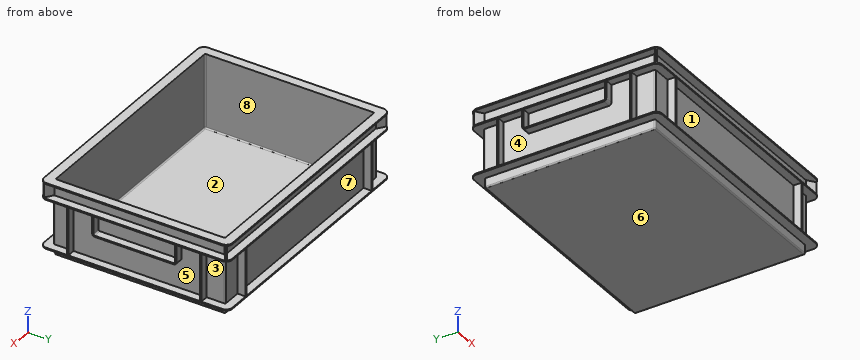
from build123d import *

# Parameters (mm, degrees)
F0_W      = 372
F0_H      = 272
F1_DEPTH  = 15
F2_W      = 372
F2_H      = 272
F3_DEPTH  = 2
F5_DEPTH  = 76
F7_DEPTH  = 2
F9_DEPTH  = 23
F11_DEPTH = 2
F12_W     = 370
F12_H     = 270
F13_DEPTH = 118
F15_DEPTH = 13
F17_DEPTH = 13
F18_R     = 2


with BuildPart() as f1:
    # F0 (on Top) → F1 (new body)
    with BuildSketch(Plane.XY):
        Rectangle(F0_W, F0_H)
    extrude(amount=F1_DEPTH)

    # F2 (on face) → F3 (join)
    with BuildSketch(Plane.XY.offset(15)):
        with BuildLine():
            Line((-190, -150), (190, -150))
            ThreePointArc((190, -150), (197.0710678119, -147.0710678119), (200, -140))
            Line((200, -140), (200, 140))
            ThreePointArc((200, 140), (197.0710678119, 147.0710678119), (190, 150))
            Line((190, 150), (-190, 150))
            ThreePointArc((-190, 150), (-197.0710678119, 147.0710678119), (-200, 140))
            Line((-200, 140), (-200, -140))
            ThreePointArc((-200, -140), (-197.0710678119, -147.0710678119), (-190, -150))
        make_face()
        Rectangle(F2_W, F2_H, mode=Mode.SUBTRACT)
        Rectangle(F2_W, F2_H)
    extrude(amount=F3_DEPTH)

    # F4 (on face) → F5 (join)
    with BuildSketch(Plane.XY.offset(17)):
        Polygon((157, -137), (187, -137), (187, -107), (200, -107), (200, -105), (187, -105), (187, 105), (200, 105), (200, 107), (187, 107), (187, 137), (157, 137), (157, 150), (155, 150), (155, 137), (-155, 137), (-155, 150), (-157, 150), (-157, 137), (-187, 137), (-187, 107), (-200, 107), (-200, 105), (-187, 105), (-187, -105), (-200, -105), (-200, -107), (-187, -107), (-187, -137), (-157, -137), (-157, -150), (-155, -150), (-155, -137), (155, -137), (155, -150), (157, -150), align=None)
    extrude(amount=F5_DEPTH)

    # F6 (on face) → F7 (join)
    with BuildSketch(Plane.XY.offset(93)):
        with BuildLine():
            Line((190, 150), (-190, 150))
            ThreePointArc((-190, 150), (-197.0710678119, 147.0710678119), (-200, 140))
            Line((-200, 140), (-200, -140))
            ThreePointArc((-200, -140), (-197.0710678119, -147.0710678119), (-190, -150))
            Line((-190, -150), (190, -150))
            ThreePointArc((190, -150), (197.0710678119, -147.0710678119), (200, -140))
            Line((200, -140), (200, 140))
            ThreePointArc((200, 140), (197.0710678119, 147.0710678119), (190, 150))
        make_face()
    extrude(amount=F7_DEPTH)

    # F8 (on face) → F9 (join)
    with BuildSketch(Plane.XY.offset(95)):
        with BuildLine():
            Line((-185.3079227659, -137), (185.3079227659, -137))
            Line((185.3079227659, -137), (197.8531877713, -146.1909160735))
            ThreePointArc((197.8531877713, -146.1909160735), (198.4340605379, -145.3727667773), (198.9300207482, -144.5005254622))
            Line((198.9300207482, -144.5005254622), (187, -135.7603498338))
            Line((187, -135.7603498338), (187, 135.7603498338))
            Line((187, 135.7603498338), (198.9300207482, 144.5005254622))
            ThreePointArc((198.9300207482, 144.5005254622), (198.4340605379, 145.3727667773), (197.8531877713, 146.1909160735))
            Line((197.8531877713, 146.1909160735), (185.3079227659, 137))
            Line((185.3079227659, 137), (-185.3079227659, 137))
            Line((-185.3079227659, 137), (-197.8531877713, 146.1909160735))
            ThreePointArc((-197.8531877713, 146.1909160735), (-198.4340605379, 145.3727667773), (-198.9300207482, 144.5005254622))
            Line((-198.9300207482, 144.5005254622), (-187, 135.7603498338))
            Line((-187, 135.7603498338), (-187, -135.7603498338))
            Line((-187, -135.7603498338), (-198.9300207482, -144.5005254622))
            ThreePointArc((-198.9300207482, -144.5005254622), (-198.4340605379, -145.3727667773), (-197.8531877713, -146.1909160735))
            Line((-197.8531877713, -146.1909160735), (-185.3079227659, -137))
        make_face()
    extrude(amount=F9_DEPTH)

    # F10 (on face) → F11 (join)
    with BuildSketch(Plane.XY.offset(118)):
        with BuildLine():
            Line((-190, -150), (190, -150))
            ThreePointArc((190, -150), (197.0710678119, -147.0710678119), (200, -140))
            Line((200, -140), (200, 140))
            ThreePointArc((200, 140), (197.0710678119, 147.0710678119), (190, 150))
            Line((190, 150), (-190, 150))
            ThreePointArc((-190, 150), (-197.0710678119, 147.0710678119), (-200, 140))
            Line((-200, 140), (-200, -140))
            ThreePointArc((-200, -140), (-197.0710678119, -147.0710678119), (-190, -150))
        make_face()
    extrude(amount=F11_DEPTH)

    # F12 (on face) → F13 (cut)
    with BuildSketch(Plane.XY.offset(120)):
        Rectangle(F12_W, F12_H)
    extrude(amount=-F13_DEPTH, mode=Mode.SUBTRACT)

    # F14 (on face) → F15 (join, through all)
    with BuildSketch(Plane(origin=(-187, 0, 0), x_dir=(0, -1, 0), z_dir=(-1, 0, 0))):
        with BuildLine():
            Line((-63, 61), (63, 61))
            ThreePointArc((63, 61), (65.8284271247, 62.1715728753), (67, 65))
            Line((67, 65), (67, 93))
            Line((67, 93), (65, 93))
            Line((65, 93), (65, 65))
            ThreePointArc((65, 65), (64.4142135624, 63.5857864376), (63, 63))
            Line((63, 63), (-63, 63))
            ThreePointArc((-63, 63), (-64.4142135624, 63.5857864376), (-65, 65))
            Line((-65, 65), (-65, 93))
            Line((-65, 93), (-67, 93))
            Line((-67, 93), (-67, 65))
            ThreePointArc((-67, 65), (-65.8284271247, 62.1715728753), (-63, 61))
        make_face()
    extrude(amount=F15_DEPTH)

    # F16 (on face) → F17 (join, through all)
    with BuildSketch(Plane.YZ.offset(187)):
        with BuildLine():
            ThreePointArc((63, 61), (65.8284271247, 62.1715728753), (67, 65))
            Line((67, 65), (67, 93))
            Line((67, 93), (65, 93))
            Line((65, 93), (65, 65))
            ThreePointArc((65, 65), (64.4142135624, 63.5857864376), (63, 63))
            Line((63, 63), (-63, 63))
            ThreePointArc((-63, 63), (-64.4142135624, 63.5857864376), (-65, 65))
            Line((-65, 65), (-65, 93))
            Line((-65, 93), (-67, 93))
            Line((-67, 93), (-67, 65))
            ThreePointArc((-67, 65), (-65.8284271247, 62.1715728753), (-63, 61))
            Line((-63, 61), (63, 61))
        make_face()
    extrude(amount=F17_DEPTH)

    # F18
    f18_edges = [f1.edges().sort_by_distance(p)[0] for p in [
        (-185, -135, 61),
        (185, -135, 61),
        (185, 135, 61),
        (0, 135, 2),
        (185, 0, 2),
        (0, -135, 2),
        (-185, 0, 2),
        (-185, 135, 61),
        (187, -137, 55),
        (187, 137, 55),
        (-187, 137, 55),
        (-187, -137, 55),
        (186, 0, 0),
        (0, 136, 0),
        (186, 136, 7.5),
        (0, -136, 0),
        (186, -136, 7.5),
        (-186, -136, 7.5),
        (-186, 0, 0),
        (-186, 136, 7.5),
    ]]
    fillet(f18_edges, radius=F18_R)


solid = f1.part
Input: part model. Units: mm. Frame: model coordinates. Face numbers are marked on the shaded views. A direction names the side the tool comes from. Give positions to 0.01 mm unless a question says otherwise; leave off trailing zeros. Write each loop counter-clockwise with the first axis right and the second up, starting at its lowest first coordinate (ties: lowest second). Pieces come first, ordered by that corner, then holes. Notation, with made-up numbers: M -11.75,-34 L 6.25,-34 A15 cw 6.25,-8 Z; hole C 19,69.5 d8. An arc over 180 degrees is marked long. Write item = value, one per line. Start each with the question number.
1) Draft query along Y for the marked faces 6, 7 and 8. Return one class per face: +Y half, -Y half, draft (parallel to the pull), parting line (faces both ways), or undercut.
2) Reachability of the marked faces 1, 2, 3, 4 and 5 from +Z, -Z, +X, -X, +Y, -Y: full face, straight path, thin tool, end or side. Return the list, or none.
3) First-contact query: pin 1 Ø1 at (y, z) = (-117.5, 36) entering from -X; pin 2 Ø6 at (x, z) = (75, 44.5) entering from -Y; pin 3 Ø4 at (x, z) = (-191, 47.5) entering from +Y. Flat tips, straight axial feed; report the tip coordinate or a pass-through.
4) Cut plane A-A on z = 111. Return the cut outline in (x, y).
5) Material intervals for line 1 along X through (y, z) = (-108, 106.5); line 2 along Y through (x, z) = (-87, 97.5); line 3 along X through (y, z) = (37, 5), sorted ascending. Write a range as [from, to].
Solved:
q1.face_6 = draft
q1.face_7 = +Y half
q1.face_8 = undercut
q2.face_1 = -Y
q2.face_2 = +Z
q2.face_3 = +X, +Y
q2.face_4 = -X
q2.face_5 = +X
q3.pin_1 = -187
q3.pin_2 = -137
q3.pin_3 = 107
q4.outline = M -198.93,-144.5 A10 ccw -197.85,-146.19 L -185.31,-137 L 185.31,-137 L 197.85,-146.19 A10 ccw 198.93,-144.5 L 187,-135.76 L 187,135.76 L 198.93,144.5 A10 ccw 197.85,146.19 L 185.31,137 L -185.31,137 L -197.85,146.19 A10 ccw -198.93,144.5 L -187,135.76 L -187,-135.76 Z; hole M -185,-133 A2 ccw -183,-135 L 183,-135 A2 ccw 185,-133 L 185,133 A2 ccw 183,135 L -183,135 A2 ccw -185,133 Z
q5.line_1 = [-187, -185], [185, 187]
q5.line_2 = [-137, -135], [135, 137]
q5.line_3 = [-186, -185], [185, 186]
